from build123d import *

# Parameters (mm, degrees)
RESSALTO_EXTRUS_O4_START = 1.5
ESBO_O6_R                = 22.720525956
ESBO_O6_R_2              = 18.220525956
RESSALTO_EXTRUS_O4_DEPTH = 1.5


with BuildPart() as part:
    # Esboço3 → Revolução2 (revolve)
    with BuildSketch(Plane.XY, mode=Mode.PRIVATE) as revolu_o2_sk:
        Polygon((-18.220525956, -9.945843652), (-11.720525956, -9.945843652), (-11.720525956, 5.554156348), (-18.220525956, 5.554156348), (-18.220525956, 2.554156348), (-22.720525956, 2.554156348), (-22.720525956, 1.054156348), (-18.220525956, 1.054156348), align=None)
    revolve(revolu_o2_sk.sketch.rotate(Axis((0, 11.544029698, 0), (0, -1, 0)), 270), axis=Axis((0, 11.544029698, 0), (0, -1, 0)))

    # Esboço6 → Ressalto-extrusão4 (add)
    with BuildSketch(Plane.XZ.offset(-1.054156348).offset(RESSALTO_EXTRUS_O4_START)):
        with Locations(Location((0, 0, 0), (0, 0, 90))):
            Circle(ESBO_O6_R)
        with Locations(Location((0, 0, 0), (0, 0, 90))):
            Circle(ESBO_O6_R_2, mode=Mode.SUBTRACT)
    extrude(amount=-RESSALTO_EXTRUS_O4_DEPTH)


solid = part.part
Can you work these out from the model? Positions are in its coordinate system, mm. A direction names the side the tool comes from. Give positions to 0.01 mm unless a question says otherwise; leave off trailing zeros. Order: outer loops, then holes, each group sorted by start corner. A loop starts at its lowest first (then second) coordinate and runs counter-clockwise, first axis right, second up. Notation, with made-up numbers: M -13.5,40 L -2.5,40 A29 ccw -2.5,67 Z; hole C 77.5,12 d3. An arc over 180 degrees is marked long. One line per question, with ' | ' between items.
Item 1: For faces 4 (the face through (-7, 2.554, 17)), 5 (the face through (-7, -0.446, -17)), 6 (the face through (12, -9.946, 0)), which set-ups out of +Z, -Z, +X, -X, +Y, -Y let a thin tool reach every point of the face, with its end or its side?
Answer block:
face 4: +Y | face 5: -Y | face 6: +Z, -Z, +X, -X, -Y
Item 2: Please list where these lines run through material, in increasing order: L1, parallel to X at y = -2, z = 0; L2, parallel to X at y = 1.25, z = 0; L3, parallel to Z at x = 10.5, y = -7.
Answer block:
L1: x = -18.22 to -11.72, 11.72 to 18.22 | L2: x = -22.72 to -11.72, 11.72 to 22.72 | L3: z = -14.89 to -5.21, 5.21 to 14.89
Item 3: I'm going to push flat-ended pins straight in: pin 1 Ø3 at (y, z) = (-4.5, 11) entering from -X; pin 2 Ø10 at (x, z) = (-2.5, -3.5) entering from +Y; pin 3 Ø8 at (x, z) = (17.5, -15) entering from +Y; pin 4 Ø3 at (x, z) = (15.5, -16) entering from -Y. Where does each tip first touch, or does it pass through?
Answer block:
pin 1: stops at x = -15.55 | pin 2: passes through | pin 3: stops at y = 2.55 | pin 4: stops at y = -0.45
Item 4: Suppose I cut it at D-D, the plane z = -15. Write out the boundary of the cut face in (x, y), then the cut area to 3 significant figures.
Answer block:
outline: M -17.07,-0.45 L -10.34,-0.45 L -10.34,-9.95 L 10.34,-9.95 L 10.34,-0.45 L 17.07,-0.45 L 17.07,2.55 L 10.34,2.55 L 10.34,5.55 L -10.34,5.55 L -10.34,2.55 L -17.07,2.55 Z | area: 361 mm2
Item 5: Suppose I cut it at A-A, the plane z = 0. Write out the boundary of the cut face in (x, y), then the cut area to 4 significant figures.
Answer block:
outline: M -22.72,-0.45 L -18.22,-0.45 L -18.22,-9.95 L -11.72,-9.95 L -11.72,5.55 L -18.22,5.55 L -18.22,2.55 L -22.72,2.55 Z; M 11.72,-9.95 L 18.22,-9.95 L 18.22,-0.45 L 22.72,-0.45 L 22.72,2.55 L 18.22,2.55 L 18.22,5.55 L 11.72,5.55 Z | area: 228.5 mm2
Item 6: We'd pull the mould along X, two halves only. Please class faces 1 (the face through (12, 5.554, 0)), 2 (the face through (-11.62, -2.09, -1.53)), 3 (the face through (13.825, 1.033, -18.03)): released by +X, released by -X, zero draft, split by the parting line, or undercut.
Answer block:
face 1: zero draft | face 2: undercut | face 3: split by the parting line
Item 7: Suppose I cut it at B-B, the plane x = 0. Write out the boundary of the cut face in (y, z), then the cut area to 4 significant figures.
Answer block:
outline: M -9.95,-18.22 L -0.45,-18.22 L -0.45,-22.72 L 2.55,-22.72 L 2.55,-18.22 L 5.55,-18.22 L 5.55,-11.72 L -9.95,-11.72 Z; M -9.95,11.72 L 5.55,11.72 L 5.55,18.22 L 2.55,18.22 L 2.55,22.72 L -0.45,22.72 L -0.45,18.22 L -9.95,18.22 Z | area: 228.5 mm2
Item 8: Suppose I cut it at C-C, the plane y = -7.5. Write out the boundary of the cut face in (x, z).
Answer block:
outline: C 0,0 d36.44; hole C 0,0 d23.44
